Read the model definition and answer for the solid it produces. Units are mm, in the model's axes. Face numbers are marked on the shaded views. A direction names the side the tool comes from. Coordinates: 2 decimals unless noted, no trailing zeros. Loops run counter-clockwise (first coordinate to the right, second up) from the corner with the lowest first, then second, coordinate; pieces in that order, holes last. Notation, with made-up numbers: M 29.25,73.5 L 63.25,73.5 A29 cw 63.25,96.5 Z; hole C 23.25,70 d8. An arc over 180 degrees is marked long. One line per item, written item: value. Start each with the question number.
1. The part is cut by section C-C (x = 7.9). Write down the section's boundary in (y, z).
2. The part is cut by section A-A (x = 27.9). Write down the section's boundary in (y, z), then the cut area to 3 significant figures.
3. Consider probe 1 along X at (y, z) = (4.6, -3.75); probe 2 along X at (y, z) = (2.7, -3.9); probe 3 along X at (y, z) = (0.5, -1.5). Determine where each line is inside the solid, lowest interval first.
4. Flat-ended cylindrical pins translate along their axes: pin 1 (2 mm diameter, centred on x = 11.9, z = -3.9, fed in from -Y); pin 2 (1 mm diameter, centred on x = 24, z = -4, fed in from -Y); pin 3 (1.4 mm diameter, centred on x = 15.9, z = -3.9, fed in from +Y). Find the tip coordinate at first contact, or state that the pin passes through.
5. For the marked faces 5, 6 and 7, determine the directions among +Z, -Z, +X, -X, +Y, -Y from which every point of the face is accessible in a straight line to the end or side of a thin tool.
6. The part is cut by section B-B (z = -6). Write down the section's boundary in (x, y), then the cut area to 3 significant figures.
7. Determine the mould class of the marked faces 1, 2, 3 and 4 for opening direction X: +X half, -X half, draft (parallel to the pull), parting line (faces both ways), or undercut.
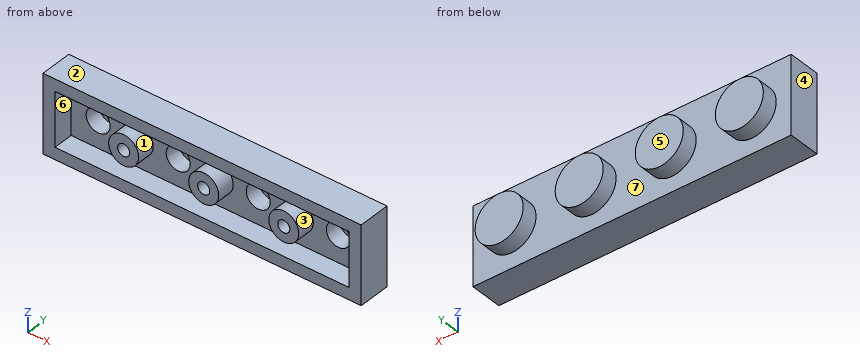
```python
from build123d import *

# Parameters (mm, degrees)
SKETCH1_W            = 31.8
SKETCH1_H            = 3.2
BOSS_EXTRUDE1_DEPTH  = 7.8
SKETCH2_R            = 2.4
BOSS_EXTRUDE2_DEPTH  = 1.6
LPATTERN1_COUNT      = 2
LPATTERN1_PITCH      = 8
LPATTERN1_COUNT_DIR2 = 6
LPATTERN1_PITCH_DIR2 = 8
SHELL1_T             = -1.2
SKETCH3_R            = 1.5
SKETCH3_R_2          = 0.6
BOSS_EXTRUDE3_DEPTH  = 1.8
LPATTERN2_COUNT      = 3
LPATTERN2_PITCH      = 8


with BuildPart() as part:
    # Sketch1 → Boss-Extrude1 (new body)
    with BuildSketch(Plane.XY):
        with Locations((15.9, 1.6)):
            Rectangle(SKETCH1_W, SKETCH1_H)
    extrude(amount=-BOSS_EXTRUDE1_DEPTH)

    # Sketch2 → Boss-Extrude2 (add)
    with BuildSketch(Plane(origin=(0, 3.2, 0), x_dir=(1, 0, 0), z_dir=(0, 1, 0))):
        with Locations(Location((3.9, 3.9, 0), (0, 0, 270))):
            Circle(SKETCH2_R)
    boss_extrude2 = extrude(amount=BOSS_EXTRUDE2_DEPTH)

    # LPattern1: Boss-Extrude2 2 × 6, 8 skipped
    with Locations(*[(j * LPATTERN1_PITCH_DIR2, 0, i * LPATTERN1_PITCH) for i in range(LPATTERN1_COUNT) for j in range(LPATTERN1_COUNT_DIR2) if (i, j) not in ((0, 0), (0, 4), (0, 5), (1, 0), (1, 1), (1, 2), (1, 3), (1, 4), (1, 5))]):
        add(boss_extrude2)

    # Shell1
    shell1_openings = [part.faces().sort_by_distance(p)[0] for p in [
        (15.9, 0, -3.9),
    ]]
    offset(amount=SHELL1_T, openings=shell1_openings, kind=Kind.INTERSECTION)

    # Sketch3 → Boss-Extrude3 (add)
    with BuildSketch(Plane.XZ.offset(-2)):
        with Locations(Location((23.9, -3.9, 0), (0, 0, 90))):
            Circle(SKETCH3_R)
        with Locations(Location((23.9, -3.9, 0), (0, 0, 270))):
            Circle(SKETCH3_R_2, mode=Mode.SUBTRACT)
    boss_extrude3 = extrude(amount=BOSS_EXTRUDE3_DEPTH)

    # LPattern2: Boss-Extrude3 ×3
    with Locations(*[(-i * LPATTERN2_PITCH, 0, 0) for i in range(1, LPATTERN2_COUNT)]):
        add(boss_extrude3)


solid = part.part
```
Answer block:
1. outline: M 0,-7.8 L 3.2,-7.8 L 3.2,0 L 0,0 L 0,-1.2 L 2,-1.2 L 2,-2.4 L 0.2,-2.4 L 0.2,-3.3 L 2,-3.3 L 2,-4.5 L 0.2,-4.5 L 0.2,-5.4 L 2,-5.4 L 2,-6.6 L 0,-6.6 Z
2. outline: M 0,-7.8 L 3.2,-7.8 L 3.2,-6.3 L 4.8,-6.3 L 4.8,-1.5 L 3.2,-1.5 L 3.2,0 L 0,0 L 0,-1.2 L 2,-1.2 L 2,-2.7 L 3.6,-2.7 L 3.6,-5.1 L 2,-5.1 L 2,-6.6 L 0,-6.6 Z
2. area: 18.0 mm2
3. probe 1: x = 1.5 to 6.3, 9.5 to 14.3, 17.5 to 22.3, 25.5 to 30.3
3. probe 2: x = 0 to 2.7, 5.1 to 10.7, 13.1 to 18.7, 21.1 to 26.7, 29.1 to 31.8
3. probe 3: x = 0 to 1.2, 30.6 to 31.8
4. pin 1: stops at y = 3.6
4. pin 2: stops at y = 0.2
4. pin 3: stops at y = 3.2
5. face 5: +Z, -Z, +X, -X, +Y
5. face 6: -Y
5. face 7: +Y
6. outline: M 0,0 L 1.2,0 L 1.2,2 L 30.6,2 L 30.6,0 L 31.8,0 L 31.8,3.2 L 29.06,3.2 L 29.06,4.8 L 26.74,4.8 L 26.74,3.2 L 21.06,3.2 L 21.06,4.8 L 18.74,4.8 L 18.74,3.2 L 13.06,3.2 L 13.06,4.8 L 10.74,4.8 L 10.74,3.2 L 5.06,3.2 L 5.06,4.8 L 2.74,4.8 L 2.74,3.2 L 0,3.2 Z
6. area: 57.8 mm2
7. face 1: undercut
7. face 2: draft
7. face 3: undercut
7. face 4: -X half
